Build history of the part. All positions in model axes, mm. A direction names the side the tool comes from. Round coordinates to 2 decimals unless told otherwise and drop trailing zeros. Loops run counter-clockwise (first coordinate to the right, second up) from the corner with the lowest first, then second, coordinate; pieces in that order, holes last. Notation, with made-up numbers: (74, -7.75) - (119, -7.75) arc R34 cw to (119, 31.25) - close; hole circle Ø4 at (-10.75, 89.25). An arc over 180 degrees is marked (long way). Use a Markdown table: item, result.
Autodesk Inventor part; units mm, degrees
ref_plane "YZ Plane" through (0, 0, 0) normal (1, 0, 0) x (0, 1, 0)
ref_plane "XZ Plane" through (0, 0, 0) normal (0, 1, 0) x (-1, 0, 0)
ref_plane "XY Plane" through (0, 0, 0) normal (0, 0, 1) x (1, 0, 0)
sketch "Sketch1" plane through (0, 0, 0) normal (0, 0, 1) x (1, 0, 0)
  circle A0 centre (0, 0) radius 6.75
  dimension "d0" = 13.5
extrude "Extrusion1" add sketch "Sketch1" along normal blind 1
sketch "Sketch2" plane through (0, 0, 1) normal (0, 0, 1) x (1, 0, 0)
  circle A0 centre (0, 0) radius 6.75
  line L0 (-6.75, 6.75) -> (6.75, 6.75) construction
  line L1 (6.75, 6.75) -> (6.75, -6.75) construction
  line L2 (6.75, -6.75) -> (-6.75, -6.75) construction
  line L3 (-6.75, -6.75) -> (-6.75, 6.75) construction
  line L4 (-6.75, 6.75) -> (6.75, -6.75) construction
  dimension "d4" = 13.5
decal "Decal1"
sketch "Sketch3" plane through (0, 0, 0) normal (0, 0, -1) x (-1, 0, 0)
  circle A0 centre (0, 0) radius 6
  dimension "d6" = 12
extrude "Extrusion2" add sketch "Sketch3" against normal blind 2.6
hole "Hole1" at (0, 0, 2.6) direction (0, 0, -1) diameter 4.8 end through all
chamfer "Chamfer1" distance 0.8 angle 45 1 edges at (0, 2.4, 2.6)
chamfer "Chamfer2" distance 0.2 angle 45 1 edges at (6, 0, 2.6)
sketch "Sketch4" plane through (0, 0, 0) normal (0, 0, -1) x (-1, 0, 0)
  circle A0 centre (0, 0) radius 2.4
  circle A1 centre (0, 0) radius 4.5
  circle A2 centre (0, 0) radius 2.4
  dimension "d24" = 9
extrude "Extrusion3" add sketch "Sketch4" along normal blind 3.9
properties part number "lens"
Q1. Cut at A-A, the plane x = 0. List the corners of the cut face in (y, z).
Results found:
| item | result |
|---|---|
| outline | (-6.75, 0) - (-4.5, 0) - (-4.5, -3.9) - (-2.4, -3.9) - (-2.4, 1.8) - (-3.2, 2.6) - (-5.8, 2.6) - (-6, 2.4) - (-6, 1) - (-6.75, 1) - close; (2.4, -3.9) - (4.5, -3.9) - (4.5, 0) - (6.75, 0) - (6.75, 1) - (6, 1) - (6, 2.4) - (5.8, 2.6) - (3.2, 2.6) - (2.4, 1.8) - close |
Q2. Which spindle directions (+Z, -Z, +X, -X, +Y, -Y) get a long thin tool onto all of the face, cutting with end or side? Do faces 1 (the face through (-1.46, 6.59, 0.49)), 2 (the face through (6, 0, 2)), 3 (the face through (4.4, 1.6, 0)). Say none if no direction does.
Results found:
| item | result |
|---|---|
| face 1 | +Z, -Z |
| face 2 | +Z |
| face 3 | -Z |
Q3. Drop flat-ended pins along their axis: pin 1 (3 mm diameter, centred on x = 4, z = -3, fed in from -Y); pin 2 (3 mm diameter, centred on x = -5.5, y = 3, fed in from -Z); pin 3 (1 mm diameter, centred on x = -0.5, z = -3, fed in from -Y). Give the stop position or say it passes through.
Results found:
| item | result |
|---|---|
| pin 1 | stops at y = -3.74 |
| pin 2 | stops at z = 0 |
| pin 3 | stops at y = -4.5 |
Q4. Probe line 1 (Y direction, x = 0, z = -1.8); line 2 (Z direction, x = -5, y = 1.5); line 3 (Z direction, x = 5, y = 4). List the from-to ranges inside material, lowest first.
Results found:
| item | result |
|---|---|
| line 1 | y = -4.5 to -2.4, 2.4 to 4.5 |
| line 2 | z = 0 to 2.6 |
| line 3 | z = 0 to 1 |
Q5. Cut at C-C, the plane z = 0.25. List the corners of the cut face in (x, y).
Results found:
| item | result |
|---|---|
| outline | circle Ø13.5 at (0, 0); hole circle Ø4.8 at (0, 0) |
